Could you check a few things on this model? Use its own coordinates, in mm. A direction names the side the tool comes from. Round coordinates to 2 decimals unless told otherwise and drop trailing zeros. Loops run counter-clockwise (first coordinate to the right, second up) from the corner with the lowest first, then second, coordinate; pieces in that order, holes last. Notation, with made-up numbers: (-17, 64) - (-8, 64) arc R27 cw to (-8, 95) - close; hole circle Ø11 at (6, 68). An arc over 180 degrees is marked (long way). Put each result on its own line as item: value. Start each with the question number.
from build123d import *

# Parameters (mm, degrees)
F0_R       = 1
F0_W       = 23
F0_H       = 12.5
F0_R_2     = 2.25
F0_W_2     = 3
F0_H_2     = 27
F1_DEPTH   = 3
F2_DEPTH   = 20
F3_SIZE2   = 24.5
F3_SIZE    = 35
F3_2_SIZE2 = 24.5
F3_2_SIZE  = 35
F4_R       = 5
F6_DEPTH   = 25
F7_DEPTH   = 2
F8_R       = 5
F9_R       = 5
F10_R      = 5
F12_DEPTH  = 25
F13_R      = 5


with BuildPart() as f1:
    # F0 (on Top) → F1 (new body)
    with BuildSketch(Plane.XY):
        with BuildLine():
            Line((-16.7032930885, 35), (-26, 35))
            Line((-26, 35), (-26, -20))
            Line((-26, -20), (-1.5, -20))
            Line((-1.5, -20), (-1.5, 7))
            Line((-1.5, 7), (1.5, 7))
            Line((1.5, 7), (1.5, -20))
            Line((1.5, -20), (26, -20))
            Line((26, -20), (26, 35))
            Line((26, 35), (16.7032930885, 35))
            ThreePointArc((16.7032930885, 35), (0, 26), (-16.7032930885, 35))
        make_face()
        with Locations((-19.375, 14)):
            Circle(F0_R, mode=Mode.SUBTRACT)
        with Locations((-5.5, 14)):
            Rectangle(F0_W, F0_H, mode=Mode.SUBTRACT)
        with Locations((8.375, 14)):
            Circle(F0_R, mode=Mode.SUBTRACT)
        with Locations((-20, 29)):
            Circle(F0_R_2, mode=Mode.SUBTRACT)
        with Locations((20, 29)):
            Circle(F0_R_2, mode=Mode.SUBTRACT)
        with Locations((0, -6.5)):
            Rectangle(F0_W_2, F0_H_2)
    extrude(amount=-F1_DEPTH)

    # F0 (on Top) → F2 (join)
    with BuildSketch(Plane.XY):
        with Locations((0, -6.5)):
            Rectangle(F0_W_2, F0_H_2)
    extrude(amount=-F2_DEPTH)

    # F3
    f3_edges = [f1.edges().sort_by_distance(p)[0] for p in [
        (-26, -20, -1.5),
    ]]
    f3_side = f1.faces().sort_by_distance((-26, 7.5, -1.5))[0]
    chamfer(f3_edges, length=F3_SIZE, length2=F3_SIZE2, reference=f3_side)

    # F3#2
    f3_2_edges = [f1.edges().sort_by_distance(p)[0] for p in [
        (26, -20, -1.5),
    ]]
    f3_2_side = f1.faces().sort_by_distance((26, 7.5, -1.5))[0]
    chamfer(f3_2_edges, length=F3_2_SIZE, length2=F3_2_SIZE2, reference=f3_2_side)

    # F4
    f4_edges = [f1.edges().sort_by_distance(p)[0] for p in [
        (-26, 35, -1.5),
        (26, 35, -1.5),
    ]]
    fillet(f4_edges, radius=F4_R)

    # F5 (on face) → F6 (cut)
    with BuildSketch(Plane(origin=(-1.5, 0, 0), x_dir=(0, -1, 0), z_dir=(-1, 0, 0))):
        with BuildLine():
            ThreePointArc((10.6381945465, -15.75), (14.5131226373, -16.2940984934), (16.625, -13))
            ThreePointArc((16.625, -13), (14.5131226373, -9.7059015066), (10.6381945465, -10.25))
            ThreePointArc((10.6381945465, -10.25), (9.375, -13), (10.6381945465, -15.75))
        make_face()
    extrude(amount=-F6_DEPTH, mode=Mode.SUBTRACT)

    # F5 (on face) → F7 (cut)
    with BuildSketch(Plane(origin=(-1.5, 0, 0), x_dir=(0, -1, 0), z_dir=(-1, 0, 0))):
        with BuildLine():
            ThreePointArc((10.6381945465, -15.75), (9.375, -13), (10.6381945465, -10.25))
            Line((10.6381945465, -10.25), (-1.3752672326, -11.0039268249))
            ThreePointArc((-1.3752672326, -11.0039268249), (0.1192088107, -11.5421703691), (0.75, -13))
            ThreePointArc((0.75, -13), (0.1192088107, -14.4578296309), (-1.3752672326, -14.9960731751))
            Line((-1.3752672326, -14.9960731751), (10.6381945465, -15.75))
        make_face()
        with BuildLine():
            ThreePointArc((0.75, -13), (0.1192088107, -11.5421703691), (-1.3752672326, -11.0039268249))
            ThreePointArc((-1.3752672326, -11.0039268249), (-3.25, -13), (-1.3752672326, -14.9960731751))
            ThreePointArc((-1.3752672326, -14.9960731751), (0.1192088107, -14.4578296309), (0.75, -13))
        make_face()
    extrude(amount=-F7_DEPTH, mode=Mode.SUBTRACT)

    # F8
    f8_edges = [f1.edges().sort_by_distance(p)[0] for p in [
        (-26, 15, -1.5),
        (26, 15, -1.5),
    ]]
    fillet(f8_edges, radius=F8_R)

    # F9
    f9_edges = [f1.edges().sort_by_distance(p)[0] for p in [
        (-16.703293, 35, -1.5),
        (16.703293, 35, -1.5),
    ]]
    fillet(f9_edges, radius=F9_R)

    # F10
    f10_edges = [f1.edges().sort_by_distance(p)[0] for p in [
        (0, -20, -20),
        (0, 7, -20),
    ]]
    fillet(f10_edges, radius=F10_R)

    # F11 (on face) → F12 (cut)
    with BuildSketch(Plane.XY):
        Polygon((7, 0.7142857143), (7, -12.1428571429), (16, 0.7142857143), align=None)
    extrude(amount=-F12_DEPTH, mode=Mode.SUBTRACT)

    # F13
    f13_edges = [f1.edges().sort_by_distance(p)[0] for p in [
        (16, 0.714286, -1.5),
        (7, 0.714286, -1.5),
        (7, -12.142857, -1.5),
    ]]
    fillet(f13_edges, radius=F13_R)


solid = f1.part
Item 1: Suppose I cut it at C-C, the plane x = 20. List the corners of the cut face in (y, z) for me, then the cut area to 3 significant figures.
Item 2: Will these pins go through, and if not, where does the flat tip stop? P1, Ø2.5, axis at x = -8, z = -1, coming from the -Y side; P2, Ø8, axis at y = 4, z = -8, coming from the -X side; P3, Ø0.9, axis at x = 0, z = -11, coming from the +Y side.
Item 3: Thinking about a two-plate mould opening in Y: for faces 4 (the face through (25, 33, -2)), 5 (the face through (-0.51, 3.25, -12.96)), 6 (the face through (0, -6, -20)), 7 (the face through (6.762, -12.09, -1.521)), which applies, released by +Y, released by -Y, zero draft, split by the parting line, or undercut?
Item 4: Suppose I cut it at B-B, the plane x = -3.5. List the corners of the cut face in (y, z) for me, then the cut area to 3 significant figures.
Item 5: On a 3-axis mill with a long thin cutter (end or side, diameter ignored), from which of +Z, -Z, +X, -X, +Y, -Y can I reach the whole of each face in a straight line? I mean faces 1 (the face through (-17.06, 34.515, -1.521)), 2 (the face through (1.5, -7, -11)), 3 (the face through (-0.514, -4.547, -15.368)). Say none if no direction works.
Item 6: Suppose I cut it at A-A, the plane z = -2. Count the separate pieces of the cut face and the enclosed holes in it, then the cut area to 3 significant figures.
Item 7: I need wall thicknesses on line 1 (X direction, y = -13, z = -6.5); line 2 (Z direction, x = -20, y = 11); line 3 (Z direction, x = -0.5, y = -7.5). Which ranges of each line are inside material? Lowest first, please. Write a range as from..to.
Numbers:
1. outline: (6.43, -3) - (26.75, -3) - (26.75, 0) - (6.43, 0) - close; (31.25, -3) - (35, -3) - (35, 0) - (31.25, 0) - close
1. area: 72.2 mm^2
2. P1: y = -12.5
2. P2: x = -1.5
2. P3: y = 7
3. face 4: released by +Y
3. face 5: undercut
3. face 6: zero draft
3. face 7: released by -Y
4. outline: (-17.14, -3) - (7.75, -3) - (7.75, 0) - (-17.14, 0) - close; (20.25, -3) - (26.31, -3) - (26.31, 0) - (20.25, 0) - close
4. area: 92.9 mm^2
5. face 1: +Z, -Z, +Y
5. face 2: -Z, +X, +Y, -Y
5. face 3: -X
6. separate pieces: 1
6. enclosed holes: 5
6. area: 1,400 mm^2
7. line 1: -1.5..1.5
7. line 2: -3..0
7. line 3: -20..-15.55, -10.45..0
